from build123d import *

# Parameters (mm, degrees)
SKETCH1_R           = 3.85
BOSS_EXTRUDE2_DEPTH = 40


with BuildPart() as part:
    # Sketch1 → Boss-Extrude2 (new body)
    # profile 1 of 2: a face of its own
    with BuildSketch(Plane(origin=(0, 0, 0), x_dir=(1, 0, 0), z_dir=(0, 1, 0))):
        with BuildLine():
            ThreePointArc((0, 5.45), (-3.853731957, 3.853731957), (-5.45, 0))
            Line((-5.45, 0), (-3.45, 0))
            ThreePointArc((-3.45, 0), (0, 3.45), (3.45, 0))
            ThreePointArc((3.45, 0), (2.439518395, -2.439518395), (0, -3.45))
            Line((0, -3.45), (0, -5.85))
            Line((0, -5.85), (5.45, -5.85))
            Line((5.45, -5.85), (14.7291644, -5.85))
            Line((14.7291644, -5.85), (14.7291644, 0.4))
            ThreePointArc((14.7291644, 0.4), (13.250053645, 3.970889245), (9.6791644, 5.45))
            Line((9.6791644, 5.45), (0, 5.45))
        make_face()
        with Locations(Location((9.6791644, 0.4, 0), (0, 0, 270))):
            Circle(SKETCH1_R, mode=Mode.SUBTRACT)
    # profile 2 of 2: a face of its own
    with BuildSketch(Plane(origin=(0, 0, 0), x_dir=(1, 0, 0), z_dir=(0, 1, 0))):
        with BuildLine():
            Line((-3.45, 0), (-5.45, 0))
            Line((-5.45, 0), (-5.45, -5.85))
            Line((-5.45, -5.85), (0, -5.85))
            Line((0, -5.85), (0, -3.45))
            ThreePointArc((0, -3.45), (-2.439518395, -2.439518395), (-3.45, 0))
        make_face()
    extrude(amount=BOSS_EXTRUDE2_DEPTH)


solid = part.part
The listing builds one solid part. Answer for the finished solid, in the listing's coordinates (mm). Give positions to 0.01 mm unless a question says otherwise; leave off trailing zeros. Write each loop counter-clockwise with the first axis right and the second up, starting at its lowest first coordinate (ties: lowest second). Pieces come first, ordered by that corner, then holes.
Item 1: Find the intervals of material crossed by line 1 along X through (y, z) = (15, -0.25); line 2 along X through (y, z) = (19.5, -1.75); line 3 along Z through (x, y) = (3, 32), in increasing order.
Item 2: A flat-ended cylindrical pin translates along its axis: P1, Ø1, axis at x = 10, z = -3, coming from the +Y side. Find the tip coordinate at first contact, or state that the pin passes through.
Item 3: Section C-C, the plane x = -1.75 is taken. Write down the section's boundary in (y, z).
Item 4: Section D-D, the plane z = 2.25 is taken. Write down the section's boundary in (x, y), plus the area to 3 significant figures.
Item 5: Determine the mould class of faces 1 (the flat face through (4, 20, 5.85)), 2 (the cylindrical face through (12.925, 19.72, 1.67)), 3 (the cylindrical face through (-3.811, 19.72, -3.896)), 4 (the cylindrical face through (13.29, 19.72, -3.93)) for opening direction X: released by +X, released by -X, zero draft, split by the parting line, or undercut.
Item 6: Section A-A, the plane y = 31 is taken. Write down the section's boundary in (x, z).
Item 7: Section B-B, the plane z = -1 is taken. Write down the section's boundary in (x, y).
Completed:
1. line 1: x = -5.44 to -3.44, 3.44 to 5.83, 13.53 to 14.73
1. line 2: x = -5.16 to -2.97, 2.97 to 6.07, 13.28 to 14.55
1. line 3: z = -5.45 to -1.7, 1.7 to 5.85
2. P1: passes through
3. outline: (0, -5.16) - (40, -5.16) - (40, -2.97) - (0, -2.97) - close; (0, 2.97) - (40, 2.97) - (40, 5.85) - (0, 5.85) - close
4. outline: (-5.45, 0) - (-2.62, 0) - (-2.62, 40) - (-5.45, 40) - close; (2.62, 0) - (6.89, 0) - (6.89, 40) - (2.62, 40) - close; (12.47, 0) - (14.73, 0) - (14.73, 40) - (12.47, 40) - close
4. area: 375 mm2
5. face 1: zero draft
5. face 2: undercut
5. face 3: released by -X
5. face 4: released by +X
6. outline: (-5.45, 0) arc R5.45 ccw to (0, -5.45) - (9.68, -5.45) arc R5.05 ccw to (14.73, -0.4) - (14.73, 5.85) - (-5.45, 5.85) - close; hole circle Ø6.9 at (0, 0); hole circle Ø7.7 at (9.68, -0.4)
7. outline: (-5.36, 0) - (-3.3, 0) - (-3.3, 40) - (-5.36, 40) - close; (3.3, 0) - (5.88, 0) - (5.88, 40) - (3.3, 40) - close; (13.48, 0) - (14.69, 0) - (14.69, 40) - (13.48, 40) - close
